```python
from build123d import *

# Parameters (mm, degrees)
F0_W     = 55
F0_H     = 30
F1_DEPTH = 3
F3_DEPTH = 100
F2_W     = 2
F2_H     = 7
F4_DEPTH = 85
F2_H_2   = 13
F5_DEPTH = 25
F6_R     = 2.25
F6_W     = 20
F6_H     = 2
F7_DEPTH = 25
F8_R     = 2.25
F9_DEPTH = 2.001


with BuildPart() as f1:
    # F0 (on Top) → F1 (new body)
    with BuildSketch(Plane.XY):
        Rectangle(F0_W, F0_H)
    extrude(amount=F1_DEPTH)

    # F2 (on face) → F3 (join)
    with BuildSketch(Plane.XY.offset(3)):
        Polygon((27.5, 15), (-27.5, 15), (-27.5, 13), (-25.5, 13), (25.5, 13), (27.5, 13), align=None)
    extrude(amount=F3_DEPTH)

    # F2 (on face) → F4 (join)
    with BuildSketch(Plane.XY.offset(3)):
        with Locations((-26.5, 9.5)):
            Rectangle(F2_W, F2_H)
        Polygon((-25.5, 6), (-27.5, 6), (-27.5, 4), (-25.5, 4), (25.5, 4), (27.5, 4), (27.5, 6), (25.5, 6), align=None)
        with Locations((26.5, 9.5)):
            Rectangle(F2_W, F2_H)
    extrude(amount=F4_DEPTH)

    # F2 (on face) → F5 (join)
    with BuildSketch(Plane.XY.offset(3)):
        with Locations((26.5, -2.5)):
            Rectangle(F2_W, F2_H_2)
        Polygon((-25.5, -9), (-27.5, -9), (-27.5, -15), (27.5, -15), (27.5, -9), (25.5, -9), align=None)
        with Locations((-26.5, -2.5)):
            Rectangle(F2_W, F2_H_2)
    extrude(amount=F5_DEPTH)

    # F6 (on face) → F7 (cut)
    with BuildSketch(Plane.XY.offset(28)):
        with Locations((0, -12)):
            Circle(F6_R)
        with Locations((6.9, -12)):
            Circle(F6_R)
        with Locations((13.8, -12)):
            Circle(F6_R)
        with Locations((20.7, -12)):
            Circle(F6_R)
        with Locations((-14.826222, -12)):
            Rectangle(F6_W, F6_H)
    extrude(amount=-F7_DEPTH, mode=Mode.SUBTRACT)

    # F8 (on face) → F9 (cut, through all)
    with BuildSketch(Plane.XZ.offset(-13)):
        with Locations((-15, 98.812126)):
            Circle(F8_R)
        with Locations((15, 98.812126)):
            Circle(F8_R)
    extrude(amount=-F9_DEPTH, mode=Mode.SUBTRACT)


solid = f1.part
```
Source: CAD feature listing. Evaluate the final solid. Frame: model axes, mm. A direction names the side the tool comes from. Give positions to 0.01 mm unless a question says otherwise; leave off trailing zeros. Order: outer loops, then holes, each group sorted by start corner. A loop starts at its lowest first (then second) coordinate and runs counter-clockwise, first axis right, second up.
(1) Pull-direction query (Z, two-part tool) for faces 4 (the face through (0, -2, 3)), 5 (the face through (5.24, -10.48, 15.68)), 6 (the face through (-15.293, 13.986, 101.043)); classes: +Z half, -Z half, draft (parallel to the pull), parting line (faces both ways), or undercut.
(2) Contact query for flat-ended pins moving along their axis: P1, Ø3, axis at x = -21, z = 77.5, coming from the -Y side; P2, Ø6, axis at x = -21, y = 6, coming from the +Z side; P3, Ø1.5, axis at x = 6, y = 1, coming from the -Z side; P4, Ø2.5, axis at x = 15, z = 98.81, coming from the +Y side. Output: stop coordinate, or through.
(3) Section query B-B (z = 70). Return the cut outline in (x, y), plus the area to 3 significant figures.
(4) Section query D-D (x = -1). Return the cut outline in (y, z), plus the area to 3 significant figures.
(5) Material intervals for line 1 along Y through (x, z) = (6.9, 14); line 2 along Y through (x, z) = (-24, 5.5); line 3 along Y through (x, z) = (-14.5, 40), sorted ascending.
(6) Section query A-A (x = -15). Return the cut outline in (y, z).
(7) Section query C-C (y = 9.75). Return the cut outline in (x, z).
(8) Access query for faces 1 (the face through (-0.13, 5.85, 88)), 2 (the face through (0, 4, 45)), 3 (the face through (14.707, 13.986, 101.043)). Directions: +Z, -Z, +X, -X, +Y, -Y. A direction counts if a zero-diameter tool reaches every point of the face in a straight line with its end or side. Return the directions, or none.
Outcome:
1. face 4: +Z half
1. face 5: draft
1. face 6: undercut
2. P1: stops at y = 4
2. P2: stops at z = 88
2. P3: stops at z = 0
2. P4: passes through
3. outline: (-27.5, 4) - (27.5, 4) - (27.5, 15) - (-27.5, 15) - close; hole (-25.5, 6) - (25.5, 6) - (25.5, 13) - (-25.5, 13) - close
3. area: 248 mm2
4. outline: (-15, 0) - (15, 0) - (15, 103) - (13, 103) - (13, 3) - (6, 3) - (6, 88) - (4, 88) - (4, 3) - (-9, 3) - (-9, 28) - (-9.98, 28) - (-9.98, 3) - (-14.02, 3) - (-14.02, 28) - (-15, 28) - close
4. area: 509 mm2
5. line 1: y = -15 to -14.25, -9.75 to -9, 4 to 6, 13 to 15
5. line 2: y = -15 to -13, -11 to -9, 4 to 6, 13 to 15
5. line 3: y = 4 to 6, 13 to 15
6. outline: (-15, 0) - (15, 0) - (15, 96.56) - (13, 96.56) - (13, 3) - (6, 3) - (6, 88) - (4, 88) - (4, 3) - (-9, 3) - (-9, 28) - (-11, 28) - (-11, 3) - (-13, 3) - (-13, 28) - (-15, 28) - close; (13, 101.06) - (15, 101.06) - (15, 103) - (13, 103) - close
7. outline: (-27.5, 0) - (27.5, 0) - (27.5, 88) - (25.5, 88) - (25.5, 3) - (-25.5, 3) - (-25.5, 88) - (-27.5, 88) - close
8. face 1: +Z, +X, -X, -Y
8. face 2: +Z
8. face 3: +Y, -Y
